Can you work these out from the drawing? Everything is in mm from the part's minimum corner. A direction names the side the tool comes from. Coordinates: 2 decimals unless noted, no trailing zeros. Loops run counter-clockwise (first coordinate to the right, second up) from the corner with the lowest first, then second, coordinate; pieces in that order, holes last.
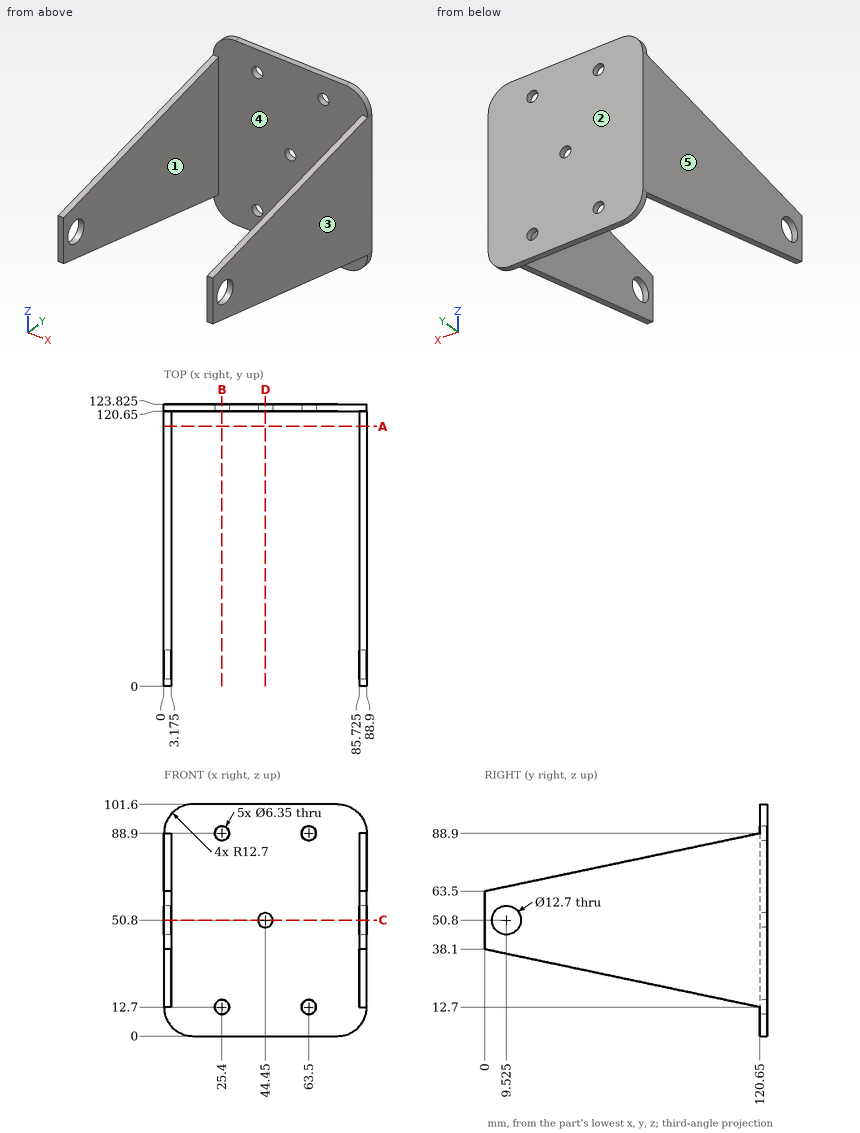
Item 1: I need wall thicknesses on line 1 along Z through (x, y) = (63.5, 121.95) (3 decimals); line 2 along X through (y, z) = (122.8, 12.7) (3 decimals); line 3 along X through (y, z) = (79.5, 50) (3 decimals). Which ranges of each line are inside material? Lowest first, please.
Results are:
line 1: z = 0 to 9.525, 15.875 to 85.725, 92.075 to 101.6
line 2: x = 0 to 22.225, 28.575 to 60.325, 66.675 to 88.9
line 3: x = 0 to 3.175, 85.725 to 88.9
Item 2: On a 3-axis mill with a long thin cutter (end or side, diameter ignored), from which of +Z, -Z, +X, -X, +Y, -Y can I reach the whole of each face in a straight line? I mean the marked faces 1 and 2. Say none if no direction works.
Results are:
face 1: +Z, -Z, -Y
face 2: +Z, -Z, +X, -X, +Y
Item 3: Suppose I cut it at B-B, the plane x = 25.4. Please give me the cut outline in (y, z) (3 decimals), plus the area to 3 significant figures.
Results are:
outline: (120.65, 0) - (123.825, 0) - (123.825, 9.525) - (120.65, 9.525) - close; (120.65, 15.875) - (123.825, 15.875) - (123.825, 85.725) - (120.65, 85.725) - close; (120.65, 92.075) - (123.825, 92.075) - (123.825, 101.6) - (120.65, 101.6) - close
area: 282 mm2
Item 4: Suppose I cut it at D-D, the plane x = 44.45. Please give me the cut outline in (y, z) (3 decimals).
Results are:
outline: (120.65, 0) - (123.825, 0) - (123.825, 47.625) - (120.65, 47.625) - close; (120.65, 53.975) - (123.825, 53.975) - (123.825, 101.6) - (120.65, 101.6) - close
Item 5: Suppose I cut it at C-C, the plane z = 50.8. Please give me the cut outline in (x, y) (3 decimals).
Results are:
outline: (0, 0) - (3.175, 0) - (3.175, 3.175) - (0, 3.175) - close; (0, 15.875) - (3.175, 15.875) - (3.175, 120.65) - (41.275, 120.65) - (41.275, 123.825) - (0, 123.825) - close; (47.625, 120.65) - (85.725, 120.65) - (85.725, 15.875) - (88.9, 15.875) - (88.9, 123.825) - (47.625, 123.825) - close; (85.725, 0) - (88.9, 0) - (88.9, 3.175) - (85.725, 3.175) - close
Item 6: I'm going to push flat-ended pins straight in: P1, Ø10, axis at x = 25.4, z = 12.7, coming from the -Y side; P2, Ø5.5, axis at x = 63.5, z = 88.9, coming from the +Y side. Where does each tip first touch, or does it pass through?
Results are:
P1: stops at y = 120.65
P2: passes through
Item 7: Suppose I cut it at A-A, the plane y = 114. Please give me the cut outline in (x, z) (3 decimals).
Results are:
outline: (0, 14.1) - (3.175, 14.1) - (3.175, 87.5) - (0, 87.5) - close; (85.725, 14.1) - (88.9, 14.1) - (88.9, 87.5) - (85.725, 87.5) - close
Item 8: We'd pull the mould along X, two halves only. Please class the marked faces 3, 4 and 5: +X half, -X half, draft (parallel to the pull), parting line (faces both ways), or undercut.
Results are:
face 3: +X half
face 4: undercut
face 5: -X half
